CAD build for the part. Positions are in the model's coordinates, mm. A direction names the side the tool comes from. Give positions to 0.01 mm unless a question says otherwise; leave off trailing zeros. Loops run counter-clockwise (first coordinate to the right, second up) from the corner with the lowest first, then second, coordinate; pieces in that order, holes last. Notation, with made-up numbers: (16.5, 57.5) -> (39.5, 57.5) arc R18 cw to (39.5, 92.5) -> close; hole circle Ø3 at (-10.5, -18). An arc over 180 degrees is marked (long way). Use one line per item in the form item = value.
```python
from build123d import *

# Parameters (mm, degrees)
BOSS_EXTRUDE1_DEPTH     = 16
SKETCH2_R               = 2
CUT_EXTRUDE1_DEPTH      = 110.166666667
CUT_EXTRUDE1_DEPTH_BACK = 321.833333333
CUT_EXTRUDE2_DEPTH      = 97.666666667


with BuildPart() as part:
    # Sketch1 → Boss-Extrude1 (new body)
    with BuildSketch(Plane.XY):
        Polygon((-96.666666667, 109.166666667), (-84.666666667, 109.166666667), (-84.666666667, -320.833333333), (-87.666666667, -320.833333333), (-87.666666667, 106.166666667), (-96.666666667, 106.166666667), align=None)
    extrude(amount=BOSS_EXTRUDE1_DEPTH)

    # Sketch2 → Cut-Extrude1 (cut, two sides)
    with BuildSketch(Plane(origin=(0, 0, 0), x_dir=(1, 0, 0), z_dir=(0, 1, 0))) as cut_extrude1_sk:
        with Locations((-92.166666667, -11.5)):
            Circle(SKETCH2_R)
        with Locations((-92.166666667, -4.5)):
            Circle(SKETCH2_R)
    extrude(amount=CUT_EXTRUDE1_DEPTH, mode=Mode.SUBTRACT)
    extrude(cut_extrude1_sk.sketch, amount=-CUT_EXTRUDE1_DEPTH_BACK, mode=Mode.SUBTRACT)

    # Sketch3 → Cut-Extrude2 (cut, through all)
    with BuildSketch(Plane(origin=(0, 0, 0), x_dir=(0, 0, -1), z_dir=(1, 0, 0))):
        with BuildLine():
            Line((-4, 89.166666667), (-4, -310.833333333))
            ThreePointArc((-4, -310.833333333), (-8, -314.833333333), (-12, -310.833333333))
            Line((-12, -310.833333333), (-12, 89.166666667))
            ThreePointArc((-12, 89.166666667), (-8, 93.166666667), (-4, 89.166666667))
        make_face()
    extrude(amount=-CUT_EXTRUDE2_DEPTH, mode=Mode.SUBTRACT)


solid = part.part
```
1. Cut at A-A, the plane y = -181.5. Write the cut outline in (x, z), then the cut area to 3 significant figures.
Result sheet:
outline = (-87.67, 0) -> (-84.67, 0) -> (-84.67, 4) -> (-87.67, 4) -> close; (-87.67, 12) -> (-84.67, 12) -> (-84.67, 16) -> (-87.67, 16) -> close
area = 24.0 mm^2
2. Tool access for faces 1 (the flat face through (-91, 109.167, 8)), 2 (the flat face through (-87.667, -110, 13)): list every direction of +Z, -Z, +X, -X, +Y, -Y with a clear straight run to the whole face (end or side of a thin tool).
Result sheet:
face_1 = +Z, -Z, +X, -X, +Y
face_2 = +Z, -Z, -X, -Y
3. Drill centre lines: line 1 (Z direction, x = -87.5, y = 72); line 2 (Y direction, x = -95, z = 14.5); line 3 (X direction, y = -71, z = 12.5). Where is each one in solid material? Low to high.
Result sheet:
line_1 = 0 to 4, 12 to 16
line_2 = 106.17 to 109.17
line_3 = -87.67 to -84.67
4. Drop flat-ended pins along their axis: P1, Ø4.5, axis at x = -94.5, z = 5, coming from the -Y side; P2, Ø6, axis at y = -234, z = 8.5, coming from the +X side. Give the stop position or say it passes through.
Result sheet:
P1 = 106.17
P2 = through
